For this review, take the finished solid that the model builds, in its own axes (mm). A direction names the side the tool comes from. Round coordinates to 2 decimals unless told otherwise and drop trailing zeros. Write each loop counter-clockwise with the first axis right and the second up, starting at its lowest first coordinate (ties: lowest second). Pieces come first, ordered by that corner, then holes.
from build123d import *

# Parameters (mm, degrees)
RESSALTO_EXTRUS_O1_DEPTH = 2.5
RESSALTO_EXTRUS_O2_DEPTH = 4
FILETE1_R                = 10
ESBO_O2_R                = 0.45
RESSALTO_EXTRUS_O3_DEPTH = 5


with BuildPart() as part:
    # Esboço1 → Ressalto-extrusão1 (new, symmetric)
    with BuildSketch(Plane(origin=(0, 0, 0), x_dir=(1, 0, 0), z_dir=(0, 1, 0))):
        with BuildLine():
            Line((-25.2, 0), (-19.2, 0))
            ThreePointArc((-19.2, 0), (-16, -3.2), (-12.8, 0))
            Line((-12.8, 0), (-11.2, 0))
            ThreePointArc((-11.2, 0), (-8, -3.2), (-4.8, 0))
            Line((-4.8, 0), (-3.2, 0))
            ThreePointArc((-3.2, 0), (0, -3.2), (3.2, 0))
            Line((3.2, 0), (4.8, 0))
            ThreePointArc((4.8, 0), (8, -3.2), (11.2, 0))
            Line((11.2, 0), (12.8, 0))
            ThreePointArc((12.8, 0), (16, -3.2), (19.2, 0))
            Line((19.2, 0), (25.2, 0))
            Line((25.2, 0), (25.2, -8.2))
            Line((25.2, -8.2), (-25.2, -8.2))
            Line((-25.2, -8.2), (-25.2, 0))
        make_face()
    extrude(amount=RESSALTO_EXTRUS_O1_DEPTH, both=True)

    # Esboço3 → Ressalto-extrusão2 (add)
    with BuildSketch(Plane(origin=(0, 2.5, 0), x_dir=(1, 0, 0), z_dir=(0, 1, 0))):
        with BuildLine():
            Line((-23.65, 5), (-23.65, 0))
            Line((-23.65, 0), (-20.75, 0))
            Line((-20.75, 0), (-20.75, 4.050862325))
            ThreePointArc((-20.75, 4.050862325), (-19.250215597, 5.474996282), (-20.7, 6.95))
            Line((-20.7, 6.95), (-21.7, 6.95))
            ThreePointArc((-21.7, 6.95), (-23.078858223, 6.378858223), (-23.65, 5))
        make_face()
        with BuildLine():
            Line((23.65, 0), (20.75, 0))
            Line((20.75, 0), (20.75, 4.050862325))
            ThreePointArc((20.75, 4.050862325), (19.250215597, 5.474996282), (20.7, 6.95))
            Line((20.7, 6.95), (21.7, 6.95))
            ThreePointArc((21.7, 6.95), (23.078858223, 6.378858223), (23.65, 5))
            Line((23.65, 5), (23.65, 0))
        make_face()
    extrude(amount=-RESSALTO_EXTRUS_O2_DEPTH)

    # Filete1
    # the kernel refuses this fillet: 10 mm, written as the material it takes off along each edge
    with BuildSketch(Plane(origin=(-25.2, 27.091665255, 8.2), x_dir=(1, 0, 0), z_dir=(0, -1, 0))) as filete1_piece_1:
        with BuildLine():
            CenterArc((9.836666102, -10), FILETE1_R, 90, 79.630240195)
            Line((0, -8.2), (-0.196733322, -8.164))
            ThreePointArc((-0.196733322, -8.164), (-0.2, -4.1), (-0.2, 0))
            Line((-0.2, 0), (0, 0.2))
            Line((0, 0.2), (9.836666102, 0.2))
            Line((9.836666102, 0.2), (9.836666102, 0))
        make_face()
    extrude(amount=54.183330509, mode=Mode.SUBTRACT)
    with BuildSketch(Plane(origin=(25.2, 27.091665255, 8.2), x_dir=(0, 0, -1), z_dir=(0, -1, 0))) as filete1_piece_2:
        with BuildLine():
            CenterArc((10, -9.836666102), FILETE1_R, 100.369759805, 79.630240195)
            Line((0, -9.836666102), (-0.2, -9.836666102))
            Line((-0.2, -9.836666102), (-0.2, 0))
            Line((-0.2, 0), (0, 0.2))
            ThreePointArc((0, 0.2), (4.1, 0.2), (8.164, 0.196733322))
            Line((8.164, 0.196733322), (8.2, 0))
        make_face()
    extrude(amount=54.183330509, mode=Mode.SUBTRACT)

    # Esboço2 → Ressalto-extrusão3 (add, through all)
    with BuildSketch(Plane(origin=(0, 2.5, 0), x_dir=(1, 0, 0), z_dir=(0, 1, 0))):
        with Locations((-12, 0)):
            Circle(ESBO_O2_R)
        with Locations((-4, 0)):
            Circle(ESBO_O2_R)
        with Locations((4, 0)):
            Circle(ESBO_O2_R)
        with Locations((12, 0)):
            Circle(ESBO_O2_R)
    extrude(amount=-RESSALTO_EXTRUS_O3_DEPTH)


solid = part.part
(1) We need section C-C, the plane z = 1.25. Give the boundary of the cut face in (x, y), and give its area (3 significant figures).
Geometry check:
outline: (-24.89, -2.5) - (-18.95, -2.5) - (-18.95, 2.5) - (-24.89, 2.5) - close; (-13.05, -2.5) - (-10.95, -2.5) - (-10.95, 2.5) - (-13.05, 2.5) - close; (-5.05, -2.5) - (-2.95, -2.5) - (-2.95, 2.5) - (-5.05, 2.5) - close; (2.95, -2.5) - (5.05, -2.5) - (5.05, 2.5) - (2.95, 2.5) - close; (10.95, -2.5) - (13.05, -2.5) - (13.05, 2.5) - (10.95, 2.5) - close; (18.95, -2.5) - (24.89, -2.5) - (24.89, 2.5) - (18.95, 2.5) - close
area: 102 mm2
(2) For line 1 along X through (y, z) = (0, -2); line 2 along X through (y, z) = (0.85, 2.75); line 3 along X through (y, z) = (0.9, 1), list the stretches that pass through material, from the lowest coordinate up.
Geometry check:
line 1: x = -23.65 to -20.75, 20.75 to 23.65
line 2: x = -24.27 to -17.64, -14.36 to -9.64, -6.36 to -1.64, 1.64 to 6.36, 9.64 to 14.36, 17.64 to 24.27
line 3: x = -24.96 to -19.04, -12.96 to -11.04, -4.96 to -3.04, 3.04 to 4.96, 11.04 to 12.96, 19.04 to 24.96
(3) For faces 4 (the face through (-19.25, 0.53, -5.44)), 5 (the face through (-22, -2, 0)), 6 (the face through (-23.65, 1, -3)), list the 3-axis set-ups (+Z, -Z, +X, -X, +Y, -Y) from which the entire face can be reached by the end or side of a thin tool; tool diameter is ignored.
Geometry check:
face 4: +Y, -Y
face 5: -Y
face 6: -Z, -X, +Y, -Y
(4) Mouldability with a two-part tool opening along Z and no side actions: class faces 1 (the face through (22, -2, 0)), 2 (the face through (-8.1, 0, 3.2)), 3 (the face through (22, -1.5, -4)) as pulls with the +Z half, pulls with the -Z half, needs draft (parallel to the pull), parting line crosses it, or undercut.
Geometry check:
face 1: undercut
face 2: pulls with the -Z half
face 3: needs draft
(5) We need section A-A, the plane z = -2.75. Give the boundary of the cut face in (x, y), and give its area (3 significant figures).
Geometry check:
outline: (-23.65, -1.5) - (-20.75, -1.5) - (-20.75, 2.5) - (-23.65, 2.5) - close; (20.75, -1.5) - (23.65, -1.5) - (23.65, 2.5) - (20.75, 2.5) - close
area: 23.2 mm2
(6) We need section D-D, the plane x = -8. Give the boundary of the cut face in (y, z), and give its area (3 significant figures).
Geometry check:
outline: (-2.5, 3.2) - (2.5, 3.2) - (2.5, 8.2) - (-2.5, 8.2) - close
area: 25.0 mm2
(7) For pin 1 Ø5 at (x, z) = (20.5, -2) entering from -Y; pin 2 Ø3 at (y, z) = (0, -3) entering from -X; pin 3 Ø5 at (x, z) = (-22, -4) entering from -Y; pin 4 Ø2 at (y, z) = (0.5, -2.5) entering from +X, all flat-tipped, find the tip position at first contact; note any pin that passes through.
Geometry check:
pin 1: stops at y = -2.5
pin 2: stops at x = -23.65
pin 3: stops at y = -1.5
pin 4: stops at x = 23.65
